from build123d import *

# Parameters (mm, degrees)
SKETCH1_W           = 66
SKETCH1_H           = 4
BOSS_EXTRUDE1_DEPTH = 90
SKETCH2_W           = 66
SKETCH2_H           = 36
BOSS_EXTRUDE2_DEPTH = 3.3
SKETCH3_W           = 66
SKETCH3_H           = 36
BOSS_EXTRUDE3_DEPTH = 3.3
SKETCH4_R           = 1.5
CUT_EXTRUDE1_DEPTH  = 104.116439039
CUT_EXTRUDE2_REACH  = 105.116
SKETCH5_W           = 18
SKETCH5_H           = 13
CUT_EXTRUDE4_REACH  = 105.116
FILLET1_R           = 2
CUT_EXTRUDE5_REACH  = 105.87
LPATTERN1_COUNT     = 5
LPATTERN1_PITCH     = 13


with BuildPart() as part:
    # Sketch1 → Boss-Extrude1 (new body)
    with BuildSketch(Plane.XY):
        Rectangle(SKETCH1_W, SKETCH1_H)
    extrude(amount=BOSS_EXTRUDE1_DEPTH)

    # Sketch2 → Boss-Extrude2 (add)
    with BuildSketch(Plane.XY.offset(90)):
        with Locations((0, -20)):
            Rectangle(SKETCH2_W, SKETCH2_H)
    extrude(amount=-BOSS_EXTRUDE2_DEPTH)

    # Sketch3 → Boss-Extrude3 (add)
    with BuildSketch(Plane(origin=(0, 0, 0), x_dir=(-1, 0, 0), z_dir=(0, 0, -1))):
        with Locations((0, -20)):
            Rectangle(SKETCH3_W, SKETCH3_H)
    extrude(amount=-BOSS_EXTRUDE3_DEPTH)

    # Sketch4 → Cut-Extrude1 (cut, through all)
    with BuildSketch(Plane.XY.offset(90)):
        with Locations((-29.5, -34)):
            Circle(SKETCH4_R)
        with Locations((29.5, -34)):
            Circle(SKETCH4_R)
    extrude(amount=-CUT_EXTRUDE1_DEPTH, mode=Mode.SUBTRACT)

    # Sketch5 → Cut-Extrude2 (cut, up to next)
    with BuildSketch(Plane.XY.offset(90), mode=Mode.PRIVATE) as cut_extrude2_sk1:
        with Locations((-15, -31.5)):
            Rectangle(SKETCH5_W, SKETCH5_H)
    cut_extrude2_tool1 = extrude(cut_extrude2_sk1.sketch, amount=-CUT_EXTRUDE2_REACH, mode=Mode.PRIVATE) & part.part
    add(cut_extrude2_tool1.solids().sort_by_distance((-15, -31.5, 90))[0], mode=Mode.SUBTRACT)

    # Sketch7 → Cut-Extrude4 (cut, up to next)
    with BuildSketch(Plane(origin=(0, 0, 0), x_dir=(-1, 0, 0), z_dir=(0, 0, -1)), mode=Mode.PRIVATE) as cut_extrude4_sk1:
        with BuildLine():
            Line((-7, -38), (23, -38))
            Line((23, -38), (23, -21))
            ThreePointArc((23, -21), (22.121320344, -18.878679656), (20, -18))
            Line((20, -18), (-4, -18))
            ThreePointArc((-4, -18), (-6.121320344, -18.878679656), (-7, -21))
            Line((-7, -21), (-7, -38))
        make_face()
    cut_extrude4_tool1 = extrude(cut_extrude4_sk1.sketch, amount=-CUT_EXTRUDE4_REACH, mode=Mode.PRIVATE) & part.part
    add(cut_extrude4_tool1.solids().sort_by_distance((-8, -28.060456, 0))[0], mode=Mode.SUBTRACT)

    # Fillet1
    fillet1_edges = [part.edges().sort_by_distance(p)[0] for p in [
        (-24, -25, 88.35),
        (-6, -25, 88.35),
    ]]
    fillet(fillet1_edges, radius=FILLET1_R)

    # Sketch8 → Cut-Extrude5 (cut, up to next)
    with BuildSketch(Plane(origin=(0, 2, 0), x_dir=(1, 0, 0), z_dir=(0, 1, 0)), mode=Mode.PRIVATE) as cut_extrude5_sk1:
        with BuildLine():
            Line((-17.2, -16.6), (17, -16.6))
            ThreePointArc((17, -16.6), (17.989949494, -17.010050506), (18.4, -18))
            Line((18.4, -18), (18.4, -19.2))
            ThreePointArc((18.4, -19.2), (17.989949494, -20.189949494), (17, -20.6))
            Line((17, -20.6), (-17.2, -20.6))
            ThreePointArc((-17.2, -20.6), (-18.189949494, -20.189949494), (-18.6, -19.2))
            Line((-18.6, -19.2), (-18.6, -18))
            ThreePointArc((-18.6, -18), (-18.189949494, -17.010050506), (-17.2, -16.6))
        make_face()
    cut_extrude5_tool1 = extrude(cut_extrude5_sk1.sketch, amount=-CUT_EXTRUDE5_REACH, mode=Mode.PRIVATE) & part.part
    cut_extrude5 = cut_extrude5_tool1.solids().sort_by_distance((-0.1, 2, 18.6))[0]
    add(cut_extrude5, mode=Mode.SUBTRACT)

    # LPattern1: Cut-Extrude5 ×5
    with Locations(*[(0, 0, i * LPATTERN1_PITCH) for i in range(1, LPATTERN1_COUNT)]):
        add(cut_extrude5, mode=Mode.SUBTRACT)


solid = part.part
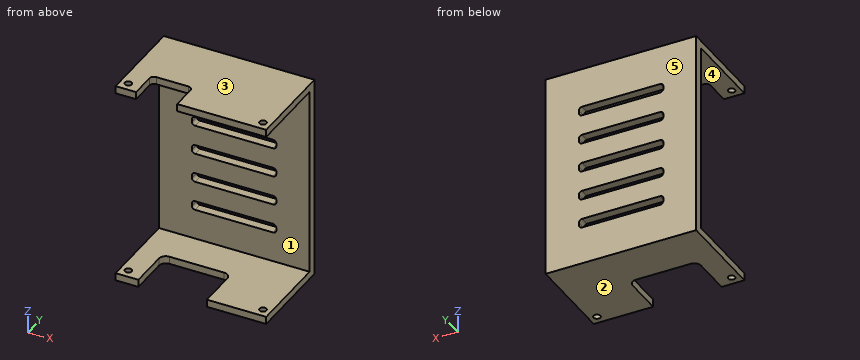
The listing builds one solid part. Answer for the finished solid, in the listing's coordinates (mm). Face numbers are marked on the shaded views. A direction names the side the tool comes from. Give positions to 0.01 mm unless a question says otherwise; leave off trailing zeros. Order: outer loops, then holes, each group sorted by start corner. A loop starts at its lowest first (then second) coordinate and runs counter-clockwise, first axis right, second up. Notation, with made-up numbers: (-10, 37.25) -> (48, 37.25) arc R25 ccw to (48, 68.25) -> close; hole circle Ø7 at (-30.75, -1.75). An arc over 180 degrees is marked (long way). Put each result on its own line as item: value.
Item 1: For the marked faces 1 and 2, determine the directions among +Z, -Z, +X, -X, +Y, -Y from which every point of the face is accessible in a straight line to the end or side of a thin tool.
Established:
face 1: +X, -X, -Y
face 2: -Z, +X, -X, +Y, -Y
Item 2: A cutting plane is placed at D-D on x = -9.5. Give the vertices of the cut face in (y, z), plus the area to 3 significant figures.
Established:
outline: (-25, 86.7) -> (-2, 86.7) -> (-2, 72.6) -> (2, 72.6) -> (2, 90) -> (-25, 90) -> close; (-18, 0) -> (2, 0) -> (2, 16.6) -> (-2, 16.6) -> (-2, 3.3) -> (-18, 3.3) -> close; (-2, 20.6) -> (2, 20.6) -> (2, 29.6) -> (-2, 29.6) -> close; (-2, 33.6) -> (2, 33.6) -> (2, 42.6) -> (-2, 42.6) -> close; (-2, 46.6) -> (2, 46.6) -> (2, 55.6) -> (-2, 55.6) -> close; (-2, 59.6) -> (2, 59.6) -> (2, 68.6) -> (-2, 68.6) -> close
area: 409 mm^2
Item 3: For a pull along Z with two mould halves and no side action, classify the marked faces 3, 4 and 5 as released by +Z, released by -Z, zero draft, split by the parting line, or undercut.
Established:
face 3: released by +Z
face 4: undercut
face 5: zero draft
Item 4: A cutting plane is placed at C-C on y = -34. Count the separate pieces of the cut face and the enclosed holes in it, plus the area to 3 significant figures.
Established:
separate pieces: 8
enclosed holes: 0
area: 238 mm^2
Item 5: Given P1, Ø8, axis at x = -10, z = 27.5, coming from the -Y side; P2, Ø2.5, axis at x = 29.5, y = -34, coming from the -Z side, each flat-ended and moving along its own axis, determine where each tip first touches the part or whether it passes through.
Established:
P1: stops at y = -2
P2: passes through
Item 6: A cutting plane is placed at B-B on y = -14.5. Give the vertices of the cut face in (x, z).
Established:
outline: (-33, 0) -> (33, 0) -> (33, 3.3) -> (-33, 3.3) -> close; (-33, 86.7) -> (33, 86.7) -> (33, 90) -> (-33, 90) -> close
Item 7: Straight lines are drawn through the part: line 1 (Y direction, x = -29.5, z = 1.5); line 2 (Z direction, x = 7, y = -10); line 3 (Z direction, x = 0.5, y = -1). For each, find the intervals that lie inside material, in ascending order.
Established:
line 1: y = -38 to -35.5, -32.5 to 2
line 2: z = 0 to 3.3, 86.7 to 90
line 3: z = 0 to 16.6, 20.6 to 29.6, 33.6 to 42.6, 46.6 to 55.6, 59.6 to 68.6, 72.6 to 90
Item 8: A cutting plane is placed at A-A on x = -29.5. Give the vertices of the cut face in (y, z).
Established:
outline: (-38, 0) -> (-35.5, 0) -> (-35.5, 3.3) -> (-38, 3.3) -> close; (-38, 86.7) -> (-35.5, 86.7) -> (-35.5, 90) -> (-38, 90) -> close; (-32.5, 0) -> (2, 0) -> (2, 90) -> (-32.5, 90) -> (-32.5, 86.7) -> (-2, 86.7) -> (-2, 3.3) -> (-32.5, 3.3) -> close
